from build123d import *

# Parameters (mm, degrees)
F0_W     = 11.1125
F0_H     = 134.9375
F0_R     = 1.7272
F1_DEPTH = 3.175
F2_R     = 3.96875
F3_R     = 3.175


with BuildPart() as f1:
    # F0 (on Top) → F1 (new body)
    with BuildSketch(Plane.XY):
        with Locations((5.55625, -67.46875)):
            Rectangle(F0_W, F0_H)
        with Locations((7.14375, -130.96875)):
            Circle(F0_R, mode=Mode.SUBTRACT)
        with Locations((7.14375, -3.96875)):
            Circle(F0_R, mode=Mode.SUBTRACT)
    extrude(amount=F1_DEPTH)

    # F2
    f2_edges = [f1.edges().sort_by_distance(p)[0] for p in [
        (11.1125, 0, 1.5875),
        (11.1125, -134.9375, 1.5875),
    ]]
    fillet(f2_edges, radius=F2_R)

    # F3
    f3_edges = [f1.edges().sort_by_distance(p)[0] for p in [
        (0, -134.9375, 1.5875),
        (0, 0, 1.5875),
    ]]
    fillet(f3_edges, radius=F3_R)


solid = f1.part
The listing builds one solid part. Answer for the finished solid, in the listing's coordinates (mm). Coordinates: 2 decimals unless noted, no trailing zeros. Answer in a Markdown table with one row per item.
1) Given pin 1 (2 mm diameter, centred on x = 7.14, y = -3.97, fed in from -Z), flat-ended and moving along its own axis, determine where the tip first touches the part or whether it passes through.
Answers below:
| item | result |
|---|---|
| pin 1 | through |
2) Determine the mould class of faces 1 (the flat face through (5, -134.938, 2)), 2 (the flat face through (0, -68, 2)), 3 (the cylindrical face through (5.87, -129.8, 1.57)) for opening direction Y: released by +Y, released by -Y, zero draft, split by the parting line, or undercut.
Answers below:
| item | result |
|---|---|
| face 1 | released by -Y |
| face 2 | zero draft |
| face 3 | undercut |
3) Find the intervals of material crossed by probe 1 along Y at (x, z) = (7, 0.4); probe 2 along Y at (x, z) = (7.75, 2.4); probe 3 along Y at (x, z) = (10.5, 1.55), in increasing order.
Answers below:
| item | result |
|---|---|
| probe 1 | -134.94 to -132.69, -129.25 to -5.69, -2.25 to 0 |
| probe 2 | -134.89 to -132.59, -129.35 to -5.59, -2.35 to -0.05 |
| probe 3 | -133.09 to -1.85 |
4) Find section A-A (z = 1.05). Count the separate pieces of the cut face and the enclosed holes in it, then the cut area to 3 significant figures.
Answers below:
| item | result |
|---|---|
| separate pieces | 1 |
| enclosed holes | 2 |
| area | 1,470 mm^2 |
